from build123d import *

# Parameters (mm, degrees)
BOSS_EXTRUDE1_DEPTH = 50.8
CUT_EXTRUDE1_REACH  = 113.741
SKETCH2_R           = 2.4
CUT_EXTRUDE2_REACH  = 115.022
SKETCH3_R           = 2.4
LPATTERN1_START     = -8.9
LPATTERN1_OUTLINE_R = 2.4
LPATTERN1_DEPTH     = 8.9


# Read off the part's stored shape, not the designer's step: LPattern1
with BuildPart() as part:
    # Sketch1 → Boss-Extrude1 (new body)
    with BuildSketch(Plane(origin=(0, 0, 0), x_dir=(0, 0, -1), z_dir=(1, 0, 0))):
        with BuildLine():
            Line((0, -25.4), (1.95, -25.4))
            Line((1.95, -25.4), (1.95, -42.683768749))
            ThreePointArc((1.95, -42.683768749), (13.853740865, -69.747329637), (41.25, -80.864))
            Line((41.25, -80.864), (41.25, -82.814))
            Line((41.25, -82.814), (66.65, -82.814))
            Line((66.65, -82.814), (66.65, -73.914))
            Line((66.65, -73.914), (41.25, -73.914))
            Line((41.25, -73.914), (41.25, -75.864))
            ThreePointArc((41.25, -75.864), (17.388850898, -66.211521802), (6.95, -42.683768749))
            Line((6.95, -42.683768749), (6.95, -25.4))
            Line((6.95, -25.4), (8.9, -25.4))
            Line((8.9, -25.4), (8.9, 0))
            Line((8.9, 0), (0, 0))
            Line((0, 0), (0, -25.4))
        make_face()
    extrude(amount=BOSS_EXTRUDE1_DEPTH)

    # Sketch2 → Cut-Extrude1 (cut, up to next)
    with BuildSketch(Plane(origin=(0, -73.914, 0), x_dir=(1, 0, 0), z_dir=(0, 1, 0)), mode=Mode.PRIVATE) as cut_extrude1_sk1:
        with Locations(Location((6.35, 60.17, 0), (0, 0, 270))):
            Circle(SKETCH2_R)
    cut_extrude1_tool1 = extrude(cut_extrude1_sk1.sketch, amount=-CUT_EXTRUDE1_REACH, mode=Mode.PRIVATE) & part.part
    # Sketch2 → Cut-Extrude1 (cut, up to next)
    with BuildSketch(Plane(origin=(0, -73.914, 0), x_dir=(1, 0, 0), z_dir=(0, 1, 0)), mode=Mode.PRIVATE) as cut_extrude1_sk2:
        with Locations(Location((31.75, 60.17, 0), (0, 0, 270))):
            Circle(SKETCH2_R)
    cut_extrude1_tool2 = extrude(cut_extrude1_sk2.sketch, amount=-CUT_EXTRUDE1_REACH, mode=Mode.PRIVATE) & part.part
    add(cut_extrude1_tool1.solids().sort_by_distance((6.35, -73.914, -60.17))[0], mode=Mode.SUBTRACT)
    add(cut_extrude1_tool2.solids().sort_by_distance((31.75, -73.914, -60.17))[0], mode=Mode.SUBTRACT)

    # Sketch3 → Cut-Extrude2 (cut, up to next)
    with BuildSketch(Plane(origin=(0, 0, -8.9), x_dir=(-1, 0, 0), z_dir=(0, 0, -1)), mode=Mode.PRIVATE) as cut_extrude2_sk1:
        with Locations(Location((-42.34, -7.6, 0), (0, 0, 90))):
            Circle(SKETCH3_R)
    cut_extrude2_tool1 = extrude(cut_extrude2_sk1.sketch, amount=-CUT_EXTRUDE2_REACH, mode=Mode.PRIVATE) & part.part
    add(cut_extrude2_tool1.solids().sort_by_distance((42.34, -7.6, -8.9))[0], mode=Mode.SUBTRACT)

    # LPattern1 outline → LPattern1 (cut)
    with BuildSketch(Plane.XY.offset(LPATTERN1_START)):
        with Locations((8.5, -7.6)):
            Circle(LPATTERN1_OUTLINE_R)
        with Locations((28.42, -7.6)):
            Circle(LPATTERN1_OUTLINE_R)
    extrude(amount=LPATTERN1_DEPTH, mode=Mode.SUBTRACT)


solid = part.part
Verification items for the finished model (mm, model axes). A direction names the side the tool comes from. Round coordinates to 2 decimals unless told otherwise and drop trailing zeros. Loops run counter-clockwise (first coordinate to the right, second up) from the corner with the lowest first, then second, coordinate; pieces in that order, holes last. Notation, with made-up numbers: (3, 35) - (57, 35) arc R13 cw to (57, 49) - close; hole circle Ø3 at (58, 66). An arc over 180 degrees is marked (long way). Use a Markdown table: item, result. Add a question column.
1. Gauge pin test, flat ends, axial feed: pin 1 (7.5 mm diameter, centred on x = 42.34, y = -7.6, fed in from -Z); pin 2 (8 mm diameter, centred on x = 9, z = -39, fed in from +Y); pin 3 (8 mm diameter, centred on x = 31, z = -26.5, fed in from +Y). Record the tip position at first contact, or that the pin passes through.
2. Section check A-A, the plane z = -60.17. Record the boundary of the cut face in (x, y), plus the area to 3 significant figures.
3. Section check C-C, the plane y = -37. Record the boundary of the cut face in (x, z).
4. Section check B-B, the plane x = 13.5. Record the boundary of the cut face in (y, z).
5. Release check for a two-part mould opening along X. For faces 5 (the face through (25, -75, -41.25)), 6 (the face through (26.022, -7.494, -4.512)), 7 (the face through (0, -53, -8)) record: released by +X, released by -X, zero draft, split by the parting line, or undercut.
6. Access from +Z, -Z, +X, -X, +Y, -Y to the whole of each face (thin tool, end or side, straight path). Record for faces 1 (the face through (25, -25.4, -1)), 2 (the face through (25, -73.914, -54)), 3 (the face through (25.04, -66.47, -17.66)), 4 (the face through (25, -25.4, -8)).
7. Thickness scan on probe 1 along X at (y, z) = (-78, -60); probe 2 along Z at (x, y) = (7, -34); probe 3 along Z at (x, y) = (39, -20.5). Record the ranges inside material, lowest first. Write a range as [from, to].
8. Section check D-D, the plane z = -15.5. Record the boundary of the cut face in (x, y), plus the area to 3 significant figures.
Checks:
| question | item | result |
|---|---|---|
| 1 | pin 1 | stops at z = -8.9 |
| 1 | pin 2 | stops at y = -73.91 |
| 1 | pin 3 | stops at y = -70.29 |
| 2 | outline | (0, -82.81) - (3.95, -82.81) - (3.95, -73.91) - (0, -73.91) - close; (8.75, -82.81) - (29.35, -82.81) - (29.35, -73.91) - (8.75, -73.91) - close; (34.15, -82.81) - (50.8, -82.81) - (50.8, -73.91) - (34.15, -73.91) - close |
| 2 | area | 367 mm^2 |
| 3 | outline | (0, -6.95) - (50.8, -6.95) - (50.8, -1.95) - (0, -1.95) - close |
| 4 | outline | (-82.81, -66.65) - (-73.91, -66.65) - (-73.91, -41.25) - (-75.86, -41.25) arc R34.32 cw to (-42.68, -6.95) - (-25.4, -6.95) - (-25.4, -8.9) - (0, -8.9) - (0, 0) - (-25.4, 0) - (-25.4, -1.95) - (-42.68, -1.95) arc R39.32 ccw to (-80.86, -41.25) - (-82.81, -41.25) - close |
| 5 | face 5 | zero draft |
| 5 | face 6 | undercut |
| 5 | face 7 | released by -X |
| 6 | face 1 | +Z, +X, -X, -Y |
| 6 | face 2 | -Z, +X, -X, +Y |
| 6 | face 3 | +X, -X |
| 6 | face 4 | -Z, +X, -X |
| 7 | probe 1 | x = [0, 3.96], [8.74, 29.36], [34.14, 50.8] |
| 7 | probe 2 | z = [-6.95, -1.95] |
| 7 | probe 3 | z = [-8.9, 0] |
| 8 | outline | (0, -71.26) - (50.8, -71.26) - (50.8, -64.23) - (0, -64.23) - close |
| 8 | area | 357 mm^2 |
